Geometry check sheet. Reference: the model listing, model coordinates, mm. Coordinates: 2 decimals unless noted, no trailing zeros. Write each loop counter-clockwise with the first axis right and the second up, starting at its lowest first coordinate (ties: lowest second). Pieces come first, ordered by that corner, then holes.
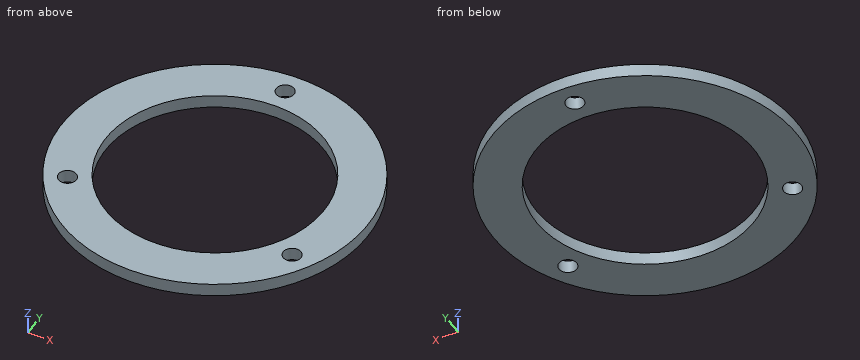
Autodesk Inventor part; units mm, degrees
ref_plane "YZ Plane" through (0, 0, 0) normal (1, 0, 0) x (0, 1, 0)
ref_plane "XZ Plane" through (0, 0, 0) normal (0, 1, 0) x (-1, 0, 0)
ref_plane "XY Plane" through (0, 0, 0) normal (0, 0, 1) x (1, 0, 0)
sketch "Sketch1" plane through (0, 0, 0) normal (0, 0, 1) x (1, 0, 0)
  circle A0 centre (0, 0) radius 25
  circle A1 centre (0, 0) radius 35
  circle A2 centre (0, 30) radius 2.05
  circle A3 centre (-25.981, -15) radius 2.05
  circle A4 centre (25.981, -15) radius 2.05
  dimension "d0" = 50
  dimension "d1" = 70
  dimension "d2" = 4.1
  dimension "d3" = 30
  dimension "d4" = 4.1
  dimension "d5" = 4.1
  dimension "d6" = 15
  dimension "d7" = 25.981
  dimension "d8" = 25.981
extrude "Extrusion1" add sketch "Sketch1" along normal blind 3
properties part number "Griff_Ring"
1. Thickness scan on line 1 along Y through (x, z) = (0, 1.4); line 2 along Y through (x, z) = (-1, 0.9); line 3 along Y through (x, z) = (19, 2.8). Record the ranges inside material, lowest first.
Computed values:
line 1: y = -35 to -25, 25 to 27.95, 32.05 to 35
line 2: y = -34.99 to -24.98, 24.98 to 28.21, 31.79 to 34.99
line 3: y = -29.39 to -16.25, 16.25 to 29.39
2. Sectioned sample at B-B, the plane z = 2.45. Record the boundary of the cut face in (x, y).
Computed values:
outline: circle Ø70 at (0, 0); hole circle Ø4.1 at (-25.98, -15); hole circle Ø50 at (0, 0); hole circle Ø4.1 at (0, 30); hole circle Ø4.1 at (25.98, -15)
3. Sectioned sample at C-C, the plane y = -2.5. Record the boundary of the cut face in (x, z).
Computed values:
outline: (-34.91, 0) - (-24.87, 0) - (-24.87, 3) - (-34.91, 3) - close; (24.87, 0) - (34.91, 0) - (34.91, 3) - (24.87, 3) - close
4. Gauge pin test, flat ends, axial feed: pin 1 Ø1 at (x, z) = (-10.5, 2.5) entering from +Y; pin 2 Ø1.5 at (x, z) = (9, 0.5) entering from +Y. Record the tip position at first contact, or that the pin passes through.
Computed values:
pin 1: stops at y = 33.54
pin 2: stops at y = 34.01
5. Sectioned sample at A-A, the plane x = 0. Record the boundary of the cut face in (y, z).
Computed values:
outline: (-35, 0) - (-25, 0) - (-25, 3) - (-35, 3) - close; (25, 0) - (27.95, 0) - (27.95, 3) - (25, 3) - close; (32.05, 0) - (35, 0) - (35, 3) - (32.05, 3) - close
6. Sectioned sample at D-D, the plane x = -14. Record the boundary of the cut face in (y, z).
Computed values:
outline: (-32.08, 0) - (-20.71, 0) - (-20.71, 3) - (-32.08, 3) - close; (20.71, 0) - (32.08, 0) - (32.08, 3) - (20.71, 3) - close
